Input: dimensioned drawing with shaded views. Units: mm. Origin: part minimum x, y, z. Give positions to 0.01 mm unless a question says otherwise; leave off trailing zeros. Write each loop counter-clockwise with the first axis right and the second up, starting at its lowest first coordinate (ties: lowest second). Pieces come first, ordered by that corner, then holes. Notation, with made-up numbers: (80, 15) -> (112, 15) arc R23 cw to (112, 23) -> close; hole circle Ø10 at (22.5, 58.25). An arc over 180 degrees is marked (long way). Answer as a JSON object with one key per item and string values.
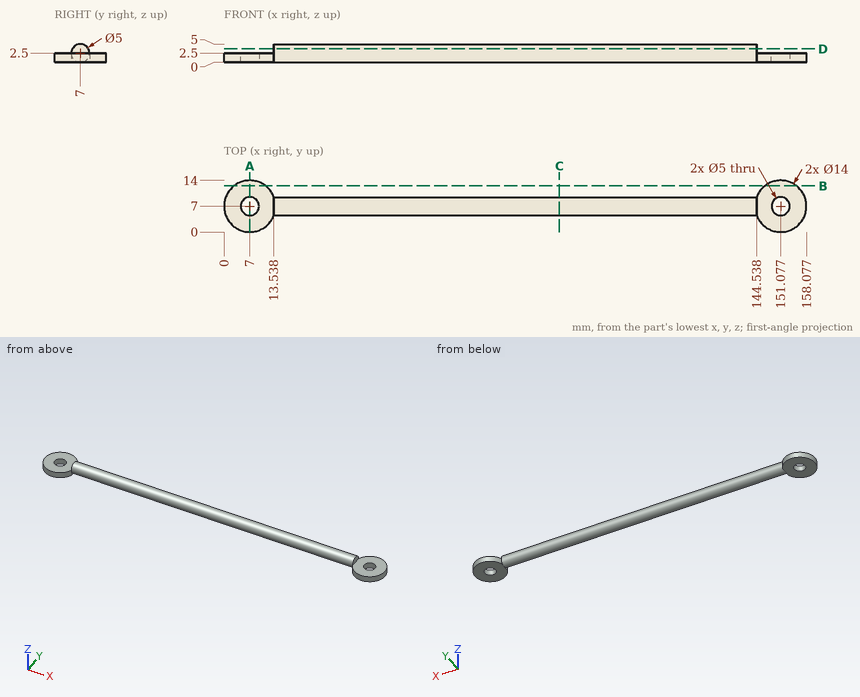
Q1. First-contact query: P1, Ø2, axis at x = 119, z = 2.5, coming from the -Y side; P2, Ø0.8, axis at y = 8, z = 4, coming from the -X side; P3, Ø1.2, axis at y = 6, z = 1.5, coming from the +X side (1 decimal); P4, Ø4, axis at x = 7, y = 7, coming from the -Z side. Flat tips, straight axial feed; report the tip coordinate or a pass-through.
Values:
{"P1": "y = 4.5", "P2": "x = 13.54", "P3": "x = 158.1", "P4": "through"}
Q2. Cut plane C-C (x = 91). Return the cut outline in (y, z).
Values:
{"outline": "circle Ø5 at (7, 2.5)"}
Q3. Material intervals for L1, parallel to X at y = 7, z = 1.85; L2, parallel to Y at x = 7, z = 1.6; L3, parallel to X at y = 7.5, z = 2.4, sorted ascending. Write a range as from..to.
Values:
{"L1": "0..4.5, 9.5..148.58, 153.58..158.08", "L2": "0..4.5, 9.5..14", "L3": "0.02..4.55, 9.45..148.63, 153.53..158.06"}
Q4. Cut plane B-B (y = 12.5). Return the cut outline in (x, z).
Values:
{"outline": "(2.67, 0) -> (11.33, 0) -> (11.33, 2.5) -> (2.67, 2.5) -> close; (146.75, 0) -> (155.41, 0) -> (155.41, 2.5) -> (146.75, 2.5) -> close"}
Q5. Cut plane A-A (x = 7). Return the cut outline in (y, z), and give its area (3 significant figures).
Values:
{"outline": "(0, 0) -> (4.5, 0) -> (4.5, 2.5) -> (0, 2.5) -> close; (9.5, 0) -> (14, 0) -> (14, 2.5) -> (9.5, 2.5) -> close", "area": "22.5 mm²"}
Q6. Cut plane D-D (z = 3.65). Return the cut outline in (x, y).
Values:
{"outline": "(13.54, 4.78) -> (144.54, 4.78) -> (144.54, 9.22) -> (13.54, 9.22) -> close"}
